The listing builds one solid part. Answer for the finished solid, in the listing's coordinates (mm). A direction names the side the tool comes from. Give positions to 0.01 mm unless a question says otherwise; leave off trailing zeros. Loops run counter-clockwise (first coordinate to the right, second up) from the corner with the lowest first, then second, coordinate; pieces in that order, holes last. Notation, with made-up numbers: M 30.5,-20 L 57.5,-20 A28 ccw 57.5,9 Z; hole C 68,-36.5 d5. An arc over 180 degrees is marked long. Return JSON: item names as keys, results as strings.
from build123d import *

# Parameters (mm, degrees)
SKETCH1_W                                         = 107.95
SKETCH1_H                                         = 101.6
BOSS_EXTRUDE1_DEPTH                               = 5.08
FILLET1_R                                         = 2.54
SKETCH2_W                                         = 98.425
SKETCH2_H                                         = 92.075
SKETCH2_W_2                                       = 92.994655172
SKETCH2_H_2                                       = 86.995
BOSS_EXTRUDE2_DEPTH                               = 2.54
SKETCH3_R                                         = 3.81
CUT_EXTRUDE1_DEPTH                                = 5.08
SKETCH4_W                                         = 6.985
SKETCH4_H                                         = 6.985
CUT_EXTRUDE2_DEPTH                                = 5.08
SKETCH5_R                                         = 2.54
CUT_EXTRUDE3_DEPTH                                = 2.54
LPATTERN1_COUNT                                   = 2
LPATTERN1_PITCH                                   = 96.52
LPATTERN1_COUNT_DIR2                              = 2
LPATTERN1_PITCH_DIR2                              = 102.87
CSK_FOR_2_FLAT_HEAD_MACHINE_SCREW_100_D           = 2.4384
CSK_FOR_2_FLAT_HEAD_MACHINE_SCREW_100_CSINK_D     = 4.3688
CSK_FOR_2_FLAT_HEAD_MACHINE_SCREW_100_CSINK_ANGLE = 100


with BuildPart() as part:
    # Sketch1 → Boss-Extrude1 (new body)
    with BuildSketch(Plane(origin=(0, 0, 0), x_dir=(1, 0, 0), z_dir=(0, 1, 0))):
        Rectangle(SKETCH1_W, SKETCH1_H)
    extrude(amount=BOSS_EXTRUDE1_DEPTH)

    # Fillet1
    fillet1_edges = [part.edges().sort_by_distance(p)[0] for p in [
        (-53.975, 5.08, 0),
        (0, 5.08, 50.8),
        (53.975, 5.08, 0),
        (0, 5.08, -50.8),
        (53.975, 2.54, 50.8),
        (-53.975, 2.54, 50.8),
        (-53.975, 2.54, -50.8),
        (53.975, 2.54, -50.8),
    ]]
    fillet(fillet1_edges, radius=FILLET1_R)

    # Sketch2 → Boss-Extrude2 (add)
    with BuildSketch(Plane.XZ):
        Rectangle(SKETCH2_W, SKETCH2_H)
        Rectangle(SKETCH2_W_2, SKETCH2_H_2, mode=Mode.SUBTRACT)
    extrude(amount=BOSS_EXTRUDE2_DEPTH)

    # Sketch3 → Cut-Extrude1 (cut)
    with BuildSketch(Plane.XZ):
        with Locations(Location((6.008676456, 29.518648142, 0), (0, 0, 270))):
            Circle(SKETCH3_R)
    extrude(amount=-CUT_EXTRUDE1_DEPTH, mode=Mode.SUBTRACT)

    # Sketch4 → Cut-Extrude2 (cut)
    with BuildSketch(Plane.XZ):
        with Locations((24.193347407, 29.518339929)):
            Rectangle(SKETCH4_W, SKETCH4_H)
    extrude(amount=-CUT_EXTRUDE2_DEPTH, mode=Mode.SUBTRACT)

    # Sketch5 → Cut-Extrude3 (cut)
    with BuildSketch(Plane(origin=(0, 5.08, 0), x_dir=(1, 0, 0), z_dir=(0, 1, 0))):
        with Locations((-51.435, -48.26)):
            Circle(SKETCH5_R)
    cut_extrude3 = extrude(amount=-CUT_EXTRUDE3_DEPTH, mode=Mode.SUBTRACT)

    # LPattern1: Cut-Extrude3 2 × 2
    with Locations(*[(j * LPATTERN1_PITCH_DIR2, 0, -i * LPATTERN1_PITCH) for i in range(LPATTERN1_COUNT) for j in range(LPATTERN1_COUNT_DIR2) if (i, j) != (0, 0)]):
        add(cut_extrude3, mode=Mode.SUBTRACT)

    # CSK for #2 Flat Head Machine Screw (100)1 (through all)
    with Locations(Plane(origin=(0, 2.54, 0), x_dir=(1, 0, 0), z_dir=(0, 1, 0))):
        with Locations((51.435, -48.26), (-51.435, -48.26), (-51.435, 48.26), (51.435, 48.26)):
            CounterSinkHole(CSK_FOR_2_FLAT_HEAD_MACHINE_SCREW_100_D / 2, CSK_FOR_2_FLAT_HEAD_MACHINE_SCREW_100_CSINK_D / 2, counter_sink_angle=CSK_FOR_2_FLAT_HEAD_MACHINE_SCREW_100_CSINK_ANGLE)


solid = part.part
(1) The part is cut by section B-B (z = 22.5). Determine the outline of the cut face in (x, y) (1 decimal).
Values follow:
{"outline": "M -54,0 L -49.2,0 L -49.2,-2.5 L -46.5,-2.5 L -46.5,0 L 46.5,0 L 46.5,-2.5 L 49.2,-2.5 L 49.2,0 L 54,0 L 54,2.5 A2.5 ccw 51.4,5.1 L -51.4,5.1 A2.5 ccw -54,2.5 Z"}
(2) Straight lines are drawn through the part: line 1 along X through (y, z) = (-0.5, 6.5); line 2 along Z through (x, y) = (44, -1.25); line 3 along X through (y, z) = (0.65, 48.26) (3 decimals). For each, find the intervals that lie inside material, in ascending order.
Values follow:
{"line 1": "-49.21 to -46.5, 46.5 to 49.21", "line 2": "-46.04 to -43.5, 43.5 to 46.04", "line 3": "-53.975 to -52.654, -50.216 to 50.216, 52.654 to 53.975"}
(3) Given pin 1 (0.8 mm diameter, centred on y = -1, z = -18.5, fed in from -X); pin 2 (1.3 mm diameter, centred on x = 10, y = -1.5, fed in from +Z); pin 3 (0.8 mm diameter, centred on y = -1, z = -22.5, fed in from +X); pin 4 (6 mm diameter, centred on x = 6.01, z = 29.52, fed in from +Y), each flat-ended and moving along its own axis, determine where each tip first touches the part or whether it passes through.
Values follow:
{"pin 1": "x = -49.21", "pin 2": "z = 46.04", "pin 3": "x = 49.21", "pin 4": "through"}
(4) A tool of negligible diameter and unlimited length cuts with its end or side. For faces 1 (the flat face through (46.497, -1, -1)), 2 (the flat face through (24, 3, 33.011)), 3 (the cylindrical face through (-49.699, 3.546, -46.406)), from which of +Z, -Z, +X, -X, +Y, -Y can it reach the whole face along a straight path? Write none if from no direction.
Values follow:
{"face 1": "-Y", "face 2": "+Y, -Y", "face 3": "+Y"}
(5) The part is cut by section A-A (x = -17). Determine the outline of the cut face in (y, z).
Values follow:
{"outline": "M -2.54,-46.04 L 0,-46.04 L 0,-50.8 L 2.54,-50.8 A2.54 ccw 5.08,-48.26 L 5.08,48.26 A2.54 ccw 2.54,50.8 L 0,50.8 L 0,46.04 L -2.54,46.04 L -2.54,43.5 L 0,43.5 L 0,-43.5 L -2.54,-43.5 Z"}
